Job drawing, mm, ordinate dimensions from the low corner. One solid piece. A direction names the side the tool comes from. Round coordinates to 2 decimals unless told otherwise and drop trailing zeros. Loops run counter-clockwise (first coordinate to the right, second up) from the corner with the lowest first, then second, coordinate; pieces in that order, holes last.
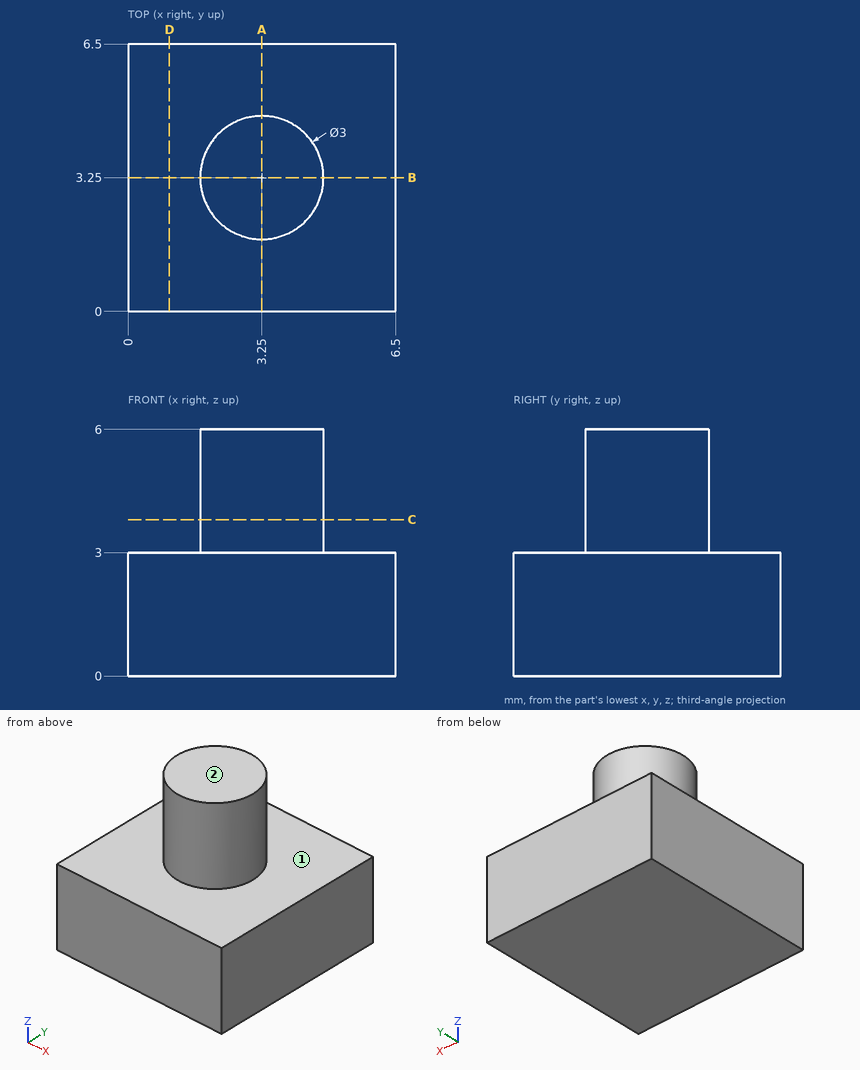
Item 1: Cut at A-A, the plane x = 3.25. Give the cut face in (y, z), plus the area to 3 significant figures.
Answers follow:
outline: (0, 0) - (6.5, 0) - (6.5, 3) - (4.75, 3) - (4.75, 6) - (1.75, 6) - (1.75, 3) - (0, 3) - close
area: 28.5 mm2
Item 2: Cut at C-C, the plane z = 3.8. Give the cut face in (x, y).
Answers follow:
outline: circle Ø3 at (3.25, 3.25)
Item 3: Cut at D-D, the plane x = 1. Give the cut face in (y, z), plus the area to 3 significant figures.
Answers follow:
outline: (0, 0) - (6.5, 0) - (6.5, 3) - (0, 3) - close
area: 19.5 mm2
Item 4: 3-axis set-ups, long thin cutter, end or side, ignore diameter. For the marked faces 1 and 2: which of +Z, -Z, +X, -X, +Y, -Y reach the whole face in a straight line?
Answers follow:
face 1: +Z
face 2: +Z, +X, -X, +Y, -Y
Item 5: Probe line 1 (Z direction, x = 1.5, y = 2.25); line 2 (Y direction, x = 2, z = 5.2); line 3 (Y direction, x = 2.5, z = 4.35). List the from-to ranges inside material, lowest first.
Answers follow:
line 1: z = 0 to 3
line 2: y = 2.42 to 4.08
line 3: y = 1.95 to 4.55
